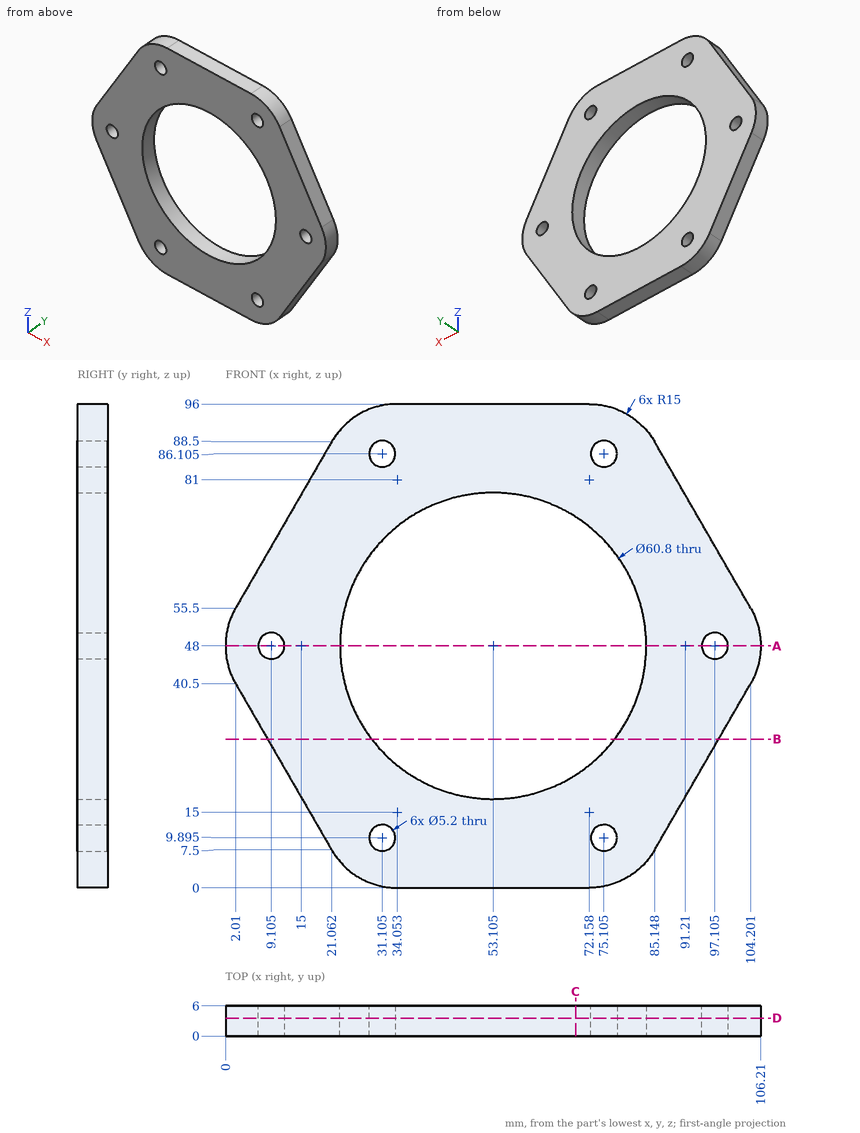
Study the drawing (mm; zero at the part's minimum x, y, z) and answer. Coordinates: 2 decimals unless noted, no trailing zeros. Order: outer loops, then holes, each group sorted by start corner. A loop starts at its lowest first (then second) coordinate and runs counter-clockwise, first axis right, second up. Notation, with made-up numbers: M 3,-5 L 23,-5 A16 cw 23,20 Z; hole C 48.25,45 d2. An arc over 180 degrees is marked long. Answer as a JSON object with one key per item and string values. Group by question number.
1. Flat-ended cylindrical pins translate along their axes: P1, Ø1, axis at y = 5, z = 41, coming from the +X side; P2, Ø4.5, axis at x = 75.11, z = 9.89, coming from the +Y side; P3, Ø1, axis at x = 89.5, y = 3, coming from the +Z side; P4, Ø3, axis at x = 32, y = 2, coming from the -Z side. Find the tip coordinate at first contact, or state that the pin passes through.
2. Section C-C on x = 69.5 is taken. Write down the section's boundary in (y, z).
3. Straight lines are drawn through the part: line 1 (Z direction, x = 53.5, y = 2.9); line 2 (X direction, y = 0.4, z = 9) (1 decimal); line 3 (Z direction, x = 37.5, y = 5.45). For each, find the intervals that lie inside material, in ascending order.
4. Section B-B on z = 29.5 is taken. Write down the section's boundary in (x, y).
5. Section A-A on z = 48 is taken. Write down the section's boundary in (x, y) (1 decimal), then the cut area to 3 significant figures.
6. Section D-D on y = 3.55 is taken. Write down the section's boundary in (x, z) (1 decimal).
Values follow:
{
 "1": {"P1": "x = 104.73", "P2": "through", "P3": "z = 81.83", "P4": "z = 0.01"},
 "2": {"outline": "M 0,0 L 6,0 L 6,22.4 L 0,22.4 Z; M 0,73.6 L 6,73.6 L 6,96 L 0,96 Z"},
 "3": {"line 1": "0 to 17.6, 78.4 to 96", "line 2": "20.2 to 28.7, 33.5 to 72.7, 77.5 to 86", "line 3": "0 to 21.91, 74.09 to 96"},
 "4": {"outline": "M 8.36,0 L 28.98,0 L 28.98,6 L 8.36,6 Z; M 77.23,0 L 97.85,0 L 97.85,6 L 77.23,6 Z"},
 "5": {"outline": "M 0,0 L 6.5,0 L 6.5,6 L 0,6 Z; M 11.7,0 L 22.7,0 L 22.7,6 L 11.7,6 Z; M 83.5,0 L 94.5,0 L 94.5,6 L 83.5,6 Z; M 99.7,0 L 106.2,0 L 106.2,6 L 99.7,6 Z", "area": "210 mm2"},
 "6": {"outline": "M 2,40.5 L 21.1,7.5 A15 ccw 34.1,0 L 72.2,0 A15 ccw 85.1,7.5 L 104.2,40.5 A15 ccw 104.2,55.5 L 85.1,88.5 A15 ccw 72.2,96 L 34.1,96 A15 ccw 21.1,88.5 L 2,55.5 A15 ccw Z; hole C 9.1,48 d5.2; hole C 53.1,48 d60.8; hole C 31.1,9.9 d5.2; hole C 31.1,86.1 d5.2; hole C 75.1,9.9 d5.2; hole C 75.1,86.1 d5.2; hole C 97.1,48 d5.2"}
}
